```python
from build123d import *

# Parameters (mm, degrees)
SALIENTE_EXTRUIR1_DEPTH = 6.35
SALIENTE_EXTRUIR2_START = -6.35
CROQUIS2_R              = 6.35
SALIENTE_EXTRUIR2_DEPTH = 6.35


with BuildPart() as part:
    # Croquis1 → Saliente-Extruir1 (new body)
    with BuildSketch(Plane(origin=(0, 0, 0), x_dir=(1, 0, 0), z_dir=(0, 1, 0))):
        with BuildLine():
            ThreePointArc((-159.524805442, 6.609301122), (-83.260417422, 44.863285815), (0, 63.5))
            ThreePointArc((0, 63.5), (44.339000485, 49.930204678), (80.270138251, 20.620826521))
            ThreePointArc((80.270138251, 20.620826521), (88.9, 0), (80.270138251, -20.620826521))
            ThreePointArc((80.270138251, -20.620826521), (44.339000485, -49.930204678), (0, -63.5))
            ThreePointArc((0, -63.5), (-83.260417422, -44.863285815), (-159.524805442, -6.609301122))
            ThreePointArc((-159.524805442, -6.609301122), (-161.925, 0), (-159.524805442, 6.609301122))
        make_face()
    extrude(amount=SALIENTE_EXTRUIR1_DEPTH)

    # Croquis2 → Saliente-Extruir2 (add)
    with BuildSketch(Plane(origin=(0, 6.35, 0), x_dir=(1, 0, 0), z_dir=(0, 1, 0)).offset(SALIENTE_EXTRUIR2_START)):
        with Locations(Location((28.575, 47.625, 0), (0, 0, 270))):
            Circle(CROQUIS2_R)
        with Locations(Location((28.575, -47.625, 0), (0, 0, 270))):
            Circle(CROQUIS2_R)
        with Locations(Location((-136.525, 0, 0), (0, 0, 270))):
            Circle(CROQUIS2_R)
    extrude(amount=-SALIENTE_EXTRUIR2_DEPTH)


solid = part.part
```
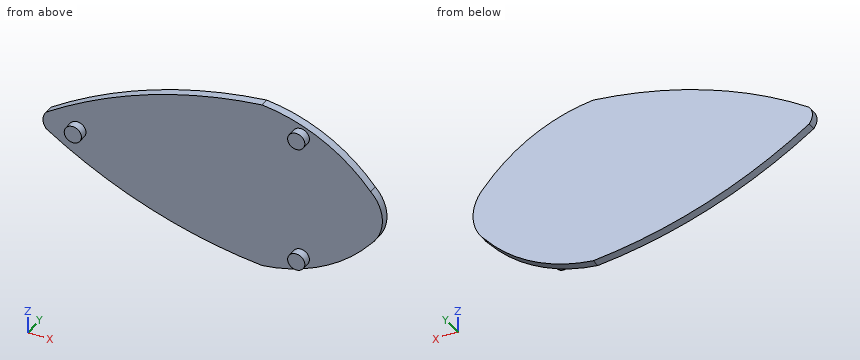
Could you check a few things on this model? Use its own coordinates, in mm. Give positions to 0.01 mm unless a question says otherwise; leave off trailing zeros. Order: outer loops, then holes, each group sorted by start corner. A loop starts at its lowest first (then second) coordinate and runs counter-clockwise, first axis right, second up.
Q1. Suppose I cut it at D-D, the plane z = -36.5. Write out the boundary of the cut face in (x, y).
Q2. If I drill on line 1 along Y through (x, z) = (71, -15); line 2 along Z through (x, y) = (-136.5, -1); line 3 along Z through (x, y) = (-2, 0.25), over which ranges is the centre line in solid material (lowest first)?
Q3. Suppose I cut it at A-A, the plane z = 0. Write out the boundary of the cut face in (x, y) (3 decimals), and give its area (3 significant figures).
Q4. I'm going to push flat-ended pins straight in: P1, Ø5, axis at x = -19, y = 2.5, coming from the -Z side; P2, Ø1, axis at x = 36.5, y = 4, coming from the -Z side; P3, Ø1.5, axis at x = -33, z = -26, coming from the -Y side. Where does each tip first touch, or does it pass through?
Q5. Suppose I cut it at B-B, the plane y = 2.5. Write out the boundary of the cut face in (x, z).
Q6. Suppose I cut it at C-C, the plane x = 11. Write out the boundary of the cut face in (y, z), and give its area (3 significant figures).
Solution:
1. outline: (-104.49, 0) - (64.36, 0) - (64.36, 6.35) - (-104.49, 6.35) - close
2. line 1: y = 0 to 6.35
2. line 2: z = -6.35 to 6.35
2. line 3: z = -63.3 to 63.3
3. outline: (-161.925, 0) - (-142.875, 0) - (-142.875, -6.35) - (-130.175, -6.35) - (-130.175, 0) - (88.9, 0) - (88.9, 6.35) - (-161.925, 6.35) - close
3. area: 1,670 mm2
4. P1: stops at z = -61.48
4. P2: stops at z = -53.98
4. P3: stops at y = 0
5. outline: (-159.52, -6.61) arc R349.52 ccw to (0, -63.5) arc R120.49 ccw to (80.27, -20.62) arc R28.95 ccw to (80.27, 20.62) arc R120.49 ccw to (0, 63.5) arc R349.52 ccw to (-159.52, 6.61) arc R10.3 ccw to start
6. outline: (0, -61.84) - (6.35, -61.84) - (6.35, 61.84) - (0, 61.84) - close
6. area: 785 mm2
